from build123d import *

# Parameters (mm, degrees)
F1_DEPTH = 571
F3_DEPTH = 25


with BuildPart() as f1:
    # F0 (on Top) → F1 (new body)
    with BuildSketch(Plane.XY):
        Polygon((40, 0), (0, 0), (0, -14), (5, -19), (25, -19), (40, -11), align=None)
    extrude(amount=F1_DEPTH)

    # F2 (on Front) → F3 (cut)
    with BuildSketch(Plane.XZ):
        Polygon((40, 40), (0, 0), (40, 0), align=None)
        Polygon((0, 571), (40, 531), (40, 571), align=None)
    extrude(amount=F3_DEPTH, mode=Mode.SUBTRACT)


solid = f1.part
Work out the finished part from the listing and answer in its coordinate system (mm). Coordinates: 2 decimals unless noted, no trailing zeros. Loops run counter-clockwise (first coordinate to the right, second up) from the corner with the lowest first, then second, coordinate; pieces in that order, holes last. Notation, with made-up numbers: (71, 7) -> (130, 7) arc R20 cw to (130, 33) -> close; hole circle Ø3 at (-28, -12.5). An arc over 180 degrees is marked (long way). Write each question's results on one line, items separated by ' | '. Start each with the question number.
1) Find section B-B on z = 49.5. Determine the outline of the cut face in (x, y), then the cut area to 4 significant figures.
2) Find section C-C on y = -7. Determine the outline of the cut face in (x, z), then the cut area to 3 significant figures.
3) Find section A-A on x = 16. Determine the outline of the cut face in (y, z).
4) Flat-ended cylindrical pins translate along their axes: P1, Ø2, axis at y = -12.5, z = 80, coming from the +X side; P2, Ø6, axis at x = 31, y = -2, coming from the +Z side; P3, Ø3, axis at x = 23.5, y = -12.5, coming from the +Z side. Find the tip coordinate at first contact, or state that the pin passes through.
5) The mould has two halves that part along Y. Classify faces 1 (the flat face through (20, -9, 551)), 2 (the flat face through (32.39, -15.06, 281.85)), 3 (the flat face through (20, 0, 282)): pulls with the +Y half, pulls with the -Y half, needs draft (parallel to the pull), parting line crosses it, or undercut.
6) Consider line 1 along Y through (x, z) = (37, 494); line 2 along Y through (x, z) = (35, 230.5); line 3 along Z through (x, y) = (20.5, -9.5). Determine where each line is inside the solid, lowest interval first.
Response values:
1) outline: (0, -14) -> (5, -19) -> (25, -19) -> (40, -11) -> (40, 0) -> (0, 0) -> close | area: 687.5 mm^2
2) outline: (0, 0) -> (40, 40) -> (40, 531) -> (0, 571) -> close | area: 21,200 mm^2
3) outline: (-19, 16) -> (0, 16) -> (0, 555) -> (-19, 555) -> close
4) P1: stops at x = 39.06 | P2: stops at z = 543 | P3: stops at z = 549
5) face 1: needs draft | face 2: pulls with the -Y half | face 3: pulls with the +Y half
6) line 1: y = -12.6 to 0 | line 2: y = -13.67 to 0 | line 3: z = 20.5 to 550.5
